Autodesk Inventor part; units mm, degrees
ref_plane "YZ Plane" through (0, 0, 0) normal (1, 0, 0) x (0, 1, 0)
ref_plane "XZ Plane" through (0, 0, 0) normal (0, 1, 0) x (-1, 0, 0)
ref_plane "XY Plane" through (0, 0, 0) normal (0, 0, 1) x (1, 0, 0)
sketch "Sketch1" plane through (0, 0, 0) normal (0, 0, 1) x (1, 0, 0)
  line L0 (-150, -80) -> (40, -80)
  line L1 (40, 80) -> (-150, 80)
  line L2 (-150, 80) -> (-150, -80)
  line L3 (-150, 0) -> (-107, 0) construction
  line L4 (-107, 0) -> (33.79, 0) construction
  line L5 (33.79, -40.6) -> (33.79, 40.6) construction
  line L6 (-6.81, 0) -> (74.39, 0) construction
  line L7 (33.79, 40.6) -> (74.39, 40.6) construction
  line L8 (74.39, 40.6) -> (74.39, 0) construction
  circle A0 centre (74.39, 40.6) radius 2
  circle A1 centre (74.39, -40.6) radius 2
  circle A2 centre (-6.81, 40.6) radius 2
  circle A3 centre (-6.81, -40.6) radius 2
  line L9 (33.79, 0) -> (33.79, 47) construction
  line L10 (33.79, 0) -> (33.79, -47) construction
  line L11 (-107, -80) -> (-107, -42.5) construction
  line L12 (-107, -42.5) -> (-71.7142, -42.5) construction
  line L13 (33.79, 0) -> (-69.7142, -42.5) construction
  circle A4 centre (-69.7142, -42.5) radius 11 construction
  line L14 (150, 0) -> (120, 0) construction
  line L15 (120, 0) -> (120, 0)
  arc A5 (40, -80) -> (120, 0) centre (40, 0) ccw
  arc A6 (120, 0) -> (40, 80) centre (40, 0) ccw
  line L16 (120, 0) -> (115, 0) construction
  circle A7 centre (115, 0) radius 1.5
  line L17 (40, 0) -> (96.5685, 56.5685) construction
  line L18 (96.5685, -56.5685) -> (93.033, -53.033) construction
  circle A8 centre (93.033, -53.033) radius 1.5
  line L19 (40, -80) -> (40, -75) construction
  circle A9 centre (40, -75) radius 1.5
  line L20 (40, -75) -> (-15, -75) construction
  line L21 (-15, -75) -> (-70, -75) construction
  line L22 (-150, -75) -> (-145, -75) construction
  circle A10 centre (-15, -75) radius 1.5
  circle A11 centre (-70, -75) radius 1.5
  circle A12 centre (-145, -75) radius 1.5
  circle A13 centre (-145, 0) radius 1.5
  circle A14 centre (93.033, 53.033) radius 1.5
  circle A15 centre (40, 75) radius 1.5
  circle A16 centre (-15, 75) radius 1.5
  circle A17 centre (-70, 75) radius 1.5
  circle A18 centre (-145, 75) radius 1.5
  line L23 (-145, -80) -> (-145, -75) construction
  line L24 (-150, 0) -> (-145, 0) construction
  line L25 (-71.7142, -42.5) -> (-67.7142, -42.5) construction
  line L26 (-85.2142, -42.5) -> (-54.2142, -42.5) construction
  line L27 (-69.7142, -27) -> (-69.7142, -58) construction
  line L28 (-69.7142, -27) -> (-85.2142, -27) construction
  line L29 (-85.2142, -27) -> (-85.2142, -42.5) construction
  circle A19 centre (-85.2142, -27) radius 1.5 construction
  circle A20 centre (-54.2142, -27) radius 1.5 construction
  circle A21 centre (-54.2142, -58) radius 1.5 construction
  circle A22 centre (-85.2142, -58) radius 1.5 construction
  line L30 (33.79, 0) -> (31.29, 0) construction
  line L31 (33.79, 0) -> (45.79, 0) construction
  line L32 (45.79, 0) -> (45.79, 58) construction
  circle A23 centre (45.79, 58) radius 1.1
  circle A24 centre (45.79, 65) radius 1.1
  line L33 (-83.2142, -27) -> (-87.2142, -27) construction
  arc A25 (-83.2142, -28.5) -> (-83.2142, -25.5) centre (-83.2142, -27) ccw
  line L34 (-83.2142, -28.5) -> (-87.2142, -28.5)
  line L35 (-83.2142, -25.5) -> (-87.2142, -25.5)
  arc A26 (-87.2142, -25.5) -> (-87.2142, -28.5) centre (-87.2142, -27) ccw
  circle A27 centre (-54.2142, -27) radius 1.5 construction
  line L36 (-56.2142, -27) -> (-52.2142, -27) construction
  arc A28 (-56.2142, -25.5) -> (-56.2142, -28.5) centre (-56.2142, -27) ccw
  line L37 (-56.2142, -28.5) -> (-52.2142, -28.5)
  line L38 (-56.2142, -25.5) -> (-52.2142, -25.5)
  arc A29 (-52.2142, -28.5) -> (-52.2142, -25.5) centre (-52.2142, -27) ccw
  line L39 (-69.7142, -58) -> (-85.2142, -58) construction
  circle A30 centre (-85.2142, -58) radius 1.5 construction
  circle A31 centre (-54.2142, -58) radius 1.5 construction
  line L40 (-83.2142, -58) -> (-87.2142, -58) construction
  arc A32 (-83.2142, -59.5) -> (-83.2142, -56.5) centre (-83.2142, -58) ccw
  line L41 (-83.2142, -56.5) -> (-87.2142, -56.5)
  line L42 (-83.2142, -59.5) -> (-87.2142, -59.5)
  arc A33 (-87.2142, -56.5) -> (-87.2142, -59.5) centre (-87.2142, -58) ccw
  line L43 (-56.2142, -56.5) -> (-52.2142, -56.5)
  arc A34 (-52.2142, -59.5) -> (-52.2142, -56.5) centre (-52.2142, -58) ccw
  line L44 (-56.2142, -58) -> (-52.2142, -58) construction
  circle A35 centre (-54.2142, -58) radius 1.5 construction
  line L45 (-56.2142, -59.5) -> (-52.2142, -59.5)
  arc A36 (-56.2142, -56.5) -> (-56.2142, -59.5) centre (-56.2142, -58) ccw
  arc A37 (-71.7142, -31.5) -> (-71.7142, -53.5) centre (-71.7142, -42.5) ccw
  arc A38 (-67.7142, -53.5) -> (-67.7142, -31.5) centre (-67.7142, -42.5) ccw
  line L46 (-67.7142, -31.5) -> (-71.7142, -31.5)
  line L47 (-67.7142, -53.5) -> (-71.7142, -53.5)
  circle A39 centre (-37.21, 22) radius 1.1
  circle A40 centre (-46.71, 22) radius 1.1
  circle A41 centre (-42.21, 42) radius 3.5
  circle A42 centre (33.79, 0) radius 6
  point P0 (0, 0)
  point P1 (120, -80)
  point P2 (120, 0)
  dimension "d4" = 43
  dimension "d6" = 140.79
  dimension "L_furos" = 81.2
  dimension "d9" = 81.2
  dimension "d11" = 4
  dimension "d30" = 47
  dimension "d40" = 37.5
  dimension "d45" = 111.89
  dimension "DN" = 22
  dimension "d47" = 30
  dimension "d49" = 80
  dimension "LF" = 5
  dimension "Furos" = 3
  dimension "d52" = 45
  dimension "d53" = 5
  dimension "d55" = 3
  dimension "d56" = 5
  dimension "d57" = 3
  dimension "d58" = 55
  dimension "d59" = 55
  dimension "d60" = 5
  dimension "d61" = 3
  dimension "d62" = 3
  dimension "d63" = 3
  dimension "d64" = 3
  dimension "d65" = 5
  dimension "d66" = 5
  dimension "d67" = 33.79
  dimension "d68" = 4
  dimension "d69" = 31
  dimension "d70" = 31
  dimension "FN" = 3
  dimension "d72" = 2.5
  dimension "d77" = 12
  dimension "NN" = 4
  dimension "d84" = 3
  dimension "d85" = 1.5
  dimension "d86" = 22
  dimension "d88" = 11
  dimension "d89" = 43
  dimension "d90" = 58
  dimension "d91" = 7
  dimension "d92" = 2.2
  dimension "d93" = 2.2
  dimension "d94" = 80
  dimension "d95" = 80
  dimension "d96" = 40
  dimension "d97" = 150
  dimension "d98" = 2.2
  dimension "d99" = 2.2
  dimension "d100" = 9.5
  dimension "d101" = 22
  dimension "d102" = 71
  dimension "d103" = 20
  dimension "d104" = 7
  dimension "d106" = 4.5
  dimension "d108" = 12
extrude "Extrusion1" add sketch "Sketch1" along normal blind 4 contours L2 L1 A6 A5 L0 | A23 | A24 | A39 | A40 | A41
extrude "Extrusion5" cut sketch "Sketch1" along normal up to surface (4 mm away) contours A39 | A40 | A41
fillet "Fillet1" radius 5 2 edges at (-150, -80, 2) (-150, 80, 2)
equation "\"d9\" = L_furos"
equation "\"d53\" = LF"
equation "\"d55\" = Furos"
equation "\"d56\" = LF"
equation "\"d57\" = Furos"
equation "\"d60\" = LF"
equation "\"d61\" = Furos"
equation "\"d62\" = Furos"
equation "\"d63\" = Furos"
equation "\"d64\" = Furos"
equation "\"d65\" = LF"
equation "\"d66\" = LF"
properties part number "Base_solida" material "Acrilico"
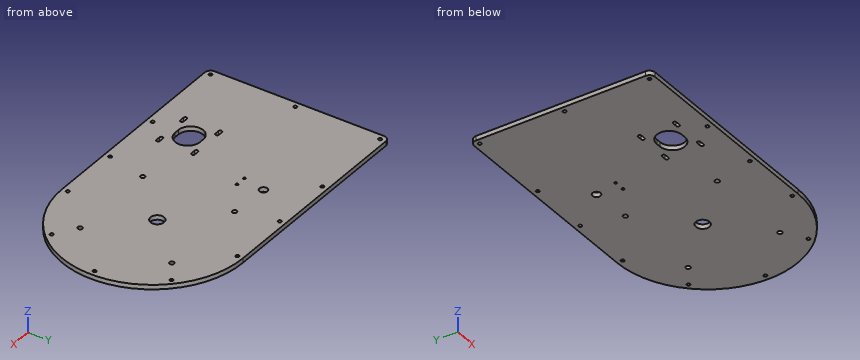
Can you work these out from the model? Positions are in its coordinate system, mm. Give positions to 0.01 mm unless a question says otherwise; leave off trailing zeros. Loops run counter-clockwise (first coordinate to the right, second up) from the corner with the lowest first, then second, coordinate; pieces in that order, holes last. Notation, with made-up numbers: M 37,84 L 84,84 A19 ccw 84,110 Z; hole C 72.5,44.5 d1. An arc over 180 degrees is marked long. Use CSV: the item, a comma, the result in double quotes. Start each with the question number.
1. If I drill on L1, parallel to Y at x = -83, z = 3.75; L2, parallel to Y at x = -15, z = 2.95; L3, parallel to Y at x = -145, z = 1.5, over which ranges is the centre line in solid material (lowest first)?
2. For P1, Ø1.5, axis at x = 64, z = 3, coming from the +Y side, with a flat end and sliding along its axis, tell me the tip position at first contact or that it passes through.
3. Imagine slicing it at C-C, the plane y = 26.5. Write out the boundary of the cut face in (x, z).
4. Imagine slicing it at A-A, the plane x = -42.21. Write out the boundary of the cut face in (y, z), plus the area to 3 significant figures.
5. Imagine slicing it at B-B, the plane y = -46.5. Write out the boundary of the cut face in (x, z).
Response values:
1,L1,"-80 to -59.48, -56.52 to -28.48, -25.52 to 80"
1,L2,"-80 to -76.5, -73.5 to 73.5, 76.5 to 80"
1,L3,"-80 to -76.5, -73.5 to -1.5, 1.5 to 73.5, 76.5 to 80"
2,P1,"y = 76.55"
3,outline,"M -150,0 L 115.48,0 L 115.48,4 L -150,4 Z"
4,outline,"M -80,0 L 38.5,0 L 38.5,4 L -80,4 Z; M 45.5,0 L 80,0 L 80,4 L 45.5,4 Z"
4,area,"612 mm^2"
5,outline,"M -150,0 L -81.96,0 L -81.96,4 L -150,4 Z; M -57.47,0 L 105.1,0 L 105.1,4 L -57.47,4 Z"
